Could you check a few things on this model? Use its own coordinates, in mm. Face numbers are marked on the shaded views. Coordinates: 2 decimals unless noted, no trailing zeros. Write each loop counter-clockwise with the first axis right and the second up, starting at its lowest first coordinate (ties: lowest second). Pieces come first, ordered by that corner, then holes.
Item 1: I want a section at A-A on y = -3.5. Please give me the cut outline in (x, z), then the cut area to 3 significant figures.
Item 2: Thinking about a two-plate mould opening in Z: for the marked faces 1, 2, 3 and 4, which applies, +Z half, -Z half, draft (parallel to the pull), parting line (faces both ways), or undercut?
Item 3: For P1, Ø1, axis at y = 5, z = 7.5, coming from the +X side; P2, Ø8, axis at x = -11.5, z = -8.5, coming from the +Y side, each with a flat end and sliding along its axis, tell me the tip position at first contact or that it passes through.
Item 4: If I drill on probe 1 along Z at (x, y) = (-0.25, -0.25); probe 2 along X at (y, z) = (4, -2.25), over which ranges is the centre line in solid material (lowest first)?
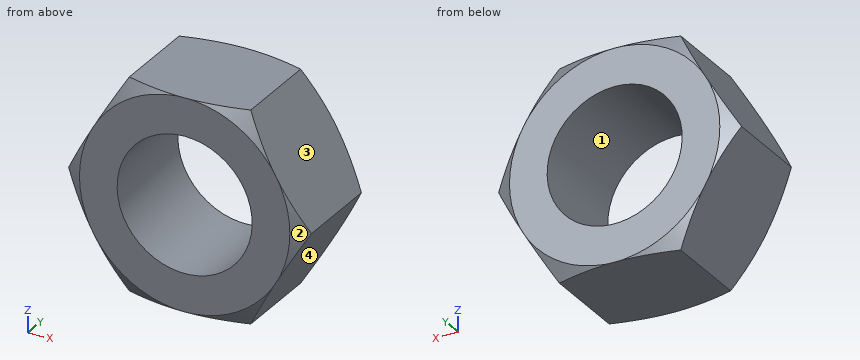
Autodesk Inventor part; units mm, degrees
ref_plane "YZ Plane" through (0, 0, 0) normal (1, 0, 0) x (0, 1, 0)
ref_plane "XZ Plane" through (0, 0, 0) normal (0, 1, 0) x (-1, 0, 0)
ref_plane "XY Plane" through (0, 0, 0) normal (0, 0, 1) x (1, 0, 0)
sketch "Sketch3" plane through (0, 0, 0) normal (0, 1, 0) x (-1, 0, 0)
  line L0 (14.6647, 0) -> (7.3323, -12.7)
  line L1 (7.3323, -12.7) -> (-7.3323, -12.7)
  line L2 (-7.3323, -12.7) -> (-14.6647, 0)
  line L3 (-14.6647, 0) -> (-7.3323, 12.7)
  line L4 (-7.3323, 12.7) -> (7.3323, 12.7)
  line L5 (7.3323, 12.7) -> (14.6647, 0)
  point P0 (0, 0)
  point P1 (0, 0)
  point P2 (0, 0)
  dimension "d27" = 25.4
extrude "Extrusion2" add sketch "Sketch3" along normal mid plane 12.7
sketch "Sketch5" plane through (0, 0, 0) normal (0, 0, 1) x (1, 0, 0)
  line L0 (0, -17.78) -> (0, 17.78)
  line L1 (14.6647, 6.35) -> (7.3323, 6.35) construction
  line L2 (7.3323, 6.35) -> (7.3323, -6.35)
  line L3 (14.6647, 6.35) -> (7.3323, 6.35)
  line L4 (14.6647, 6.35) -> (14.6647, -6.35) construction
  line L5 (7.3323, -6.35) -> (14.6647, -6.35)
  line L6 (12.7, 6.35) -> (14.6647, 6.35)
  line L7 (14.6647, 6.35) -> (14.6647, 5.2157)
  line L8 (14.6647, 5.2157) -> (12.7, 6.35)
  line L9 (0, 0) -> (14.3088, 0) construction
  line L10 (12.7, -6.35) -> (14.6647, -6.35)
  line L11 (14.6647, -6.35) -> (14.6647, -5.2157)
  line L12 (14.6647, -5.2157) -> (12.7, -6.35)
  dimension "d15" = 25.4
  dimension "d16" = 30
revolve "Revolution3" cut sketch "Sketch5" angle 360 about axis through (0, -10, 0) along (0, 1, 0)
hole "Hole1" at (0, 6.35, 0) direction (0, -1, 0) diameter 16.3068 end through all
equation "\"diameter\" = 25.4"
equation "\"length\" = 76.2"
properties part number "Hinge Pin Nut" material "Steel, Carbon"
Response values:
1. outline: (-14.66, 0) - (-7.33, -12.7) - (7.33, -12.7) - (14.66, 0) - (7.33, 12.7) - (-7.33, 12.7) - close; hole circle Ø16.31 at (0, 0)
1. area: 350 mm2
2. face 1: undercut
2. face 2: parting line
2. face 3: +Z half
2. face 4: -Z half
3. P1: stops at x = 10.62
3. P2: stops at y = 6.35
4. probe 1: z = -12.7 to -8.15, 8.15 to 12.7
4. probe 2: x = -13.37 to -7.84, 7.84 to 13.37
